```python
from build123d import *

# Parameters (mm, degrees)
THICKEN1_T1 = 10


with BuildPart() as body_1:
    # Sketch2 → Surface-Plane1: a flat surface bounded by the sketch
    with BuildSketch(Plane(origin=(0, 0, 0), x_dir=(1, 0, 0), z_dir=(0, 1, 0)), mode=Mode.PRIVATE) as surface_plane1_1_region:
        with BuildLine():
            Line((60, -101.35), (-60, -101.35))
            Line((-60, -101.35), (-60, 101.35))
            ThreePointArc((-60, 101.35), (-47.087611837, 167.497853897), (-16.523672609, 227.565432191))
            ThreePointArc((-16.523672609, 227.565432191), (-0.064821019, 236.113976909), (16.340966999, 227.464032864))
            ThreePointArc((16.340966999, 227.464032864), (46.741380265, 167.374149084), (60, 101.35))
            Line((60, 101.35), (60, -101.35))
        make_face()
    surface_plane1_1 = surface_plane1_1_region.sketch.faces()[0]
    add(Solid.thicken(surface_plane1_1, THICKEN1_T1))


solid = body_1.part
```
The model under review builds one solid part; all positions refer to its coordinate system, in mm. Round coordinates to 2 decimals unless told otherwise and drop trailing zeros. Loops run counter-clockwise (first coordinate to the right, second up) from the corner with the lowest first, then second, coordinate; pieces in that order, holes last. Notation, with made-up numbers: M 50,-7.5 L 91,-7.5 A15 ccw 91,21.5 Z; hole C 6.5,-24 d1. An arc over 180 degrees is marked long. Write item = value, one per line.
Item 1: Take a section at A-A on y = 4.5. Write out the cut boundary in (x, z), then the cut area to 3 significant figures.
Return value:
outline = M -60,-101.35 A243.3 ccw -16.52,-227.57 A20 ccw 16.34,-227.46 A250 ccw 60,-101.35 L 60,101.35 L -60,101.35 Z
area = 35,800 mm2
Item 2: Take a section at B-B on x = 44. Write out the cut boundary in (y, z).
Return value:
outline = M 0,-174.9 L 10,-174.9 L 10,101.35 L 0,101.35 Z
Item 3: Insertion check: P1, Ø4, axis at x = 36, y = 2.5, coming from the -Z side; P2, Ø5, axis at y = 7.5, z = -152, coming from the +X side. Each pin has a flat end and moves straight along its axis. Give the tip position at first contact, or say it passes through.
Return value:
P1 = -197.6
P2 = 52.19
Item 4: Take a section at C-C on z = -120. Write out the cut boundary in (x, y).
Return value:
outline = M -58.27,0 L 58.12,0 L 58.12,10 L -58.27,10 Z
Item 5: For line 1 (Z direction, x = -21.5, y = 7.5); line 2 (Z direction, x = -9, y = 1.25); line 3 (X direction, y = 7, z = -103), list the stretches that pass through material, from the lowest coordinate up. Write a range as [from, to].
Return value:
line_1 = [-220.15, 101.35]
line_2 = [-234.04, 101.35]
line_3 = [-59.91, 59.89]
